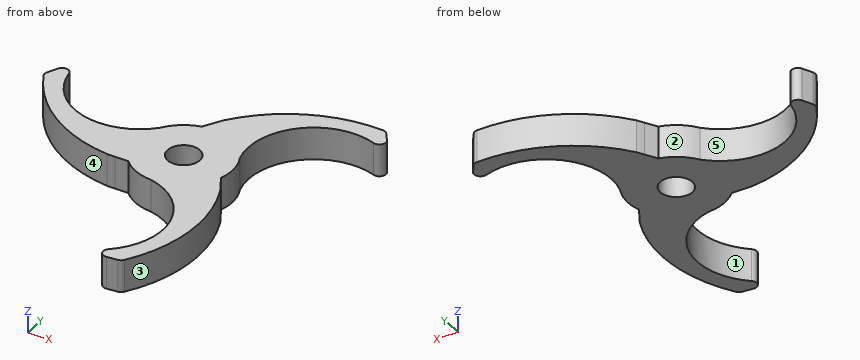
Autodesk Inventor part; units mm, degrees
ref_plane "Work Plane3" through (0, 0, 5) normal (0, 0, -1) x (-1, 0, 0)
ref_plane "YZ Plane" through (0, 0, 0) normal (1, 0, 0) x (0, 1, 0)
ref_plane "XZ Plane" through (0, 0, 0) normal (0, 1, 0) x (-1, 0, 0)
sketch "Sketch1" plane through (0, 0, 0) normal (0, 0, 1) x (1, 0, 0)
  circle A0 centre (0, 0) radius 15
  circle A1 centre (0, 0) radius 55
  line L0 (15, 0) -> (55, 0) construction
  circle A2 centre (35, 0) radius 20 construction
  circle A3 centre (-17.5, 30.3109) radius 20 construction
  circle A4 centre (-17.5, -30.3109) radius 20 construction
  line L1 (0, 0) -> (-10.834, 10.3742)
  line L2 (0, 0) -> (27.5, -47.6314)
  line L3 (0, 0) -> (-55, 0) construction
  line L4 (0, 0) -> (27.5, 47.6314)
  line L5 (17.5, 30.3109) -> (27.5, 47.6314) construction
  line L6 (-1.4324, 18.1475) -> (18.5676, 52.7885) construction
  line L7 (18.5676, 52.7885) -> (36.4324, 42.4743) construction
  line L8 (36.4324, 42.4743) -> (16.4324, 7.8333) construction
  line L9 (16.4324, 7.8333) -> (-1.4324, 18.1475) construction
  line L10 (-1.4324, 18.1475) -> (36.4324, 42.4743) construction
  line L11 (18.5676, 52.7885) -> (16.4324, 7.8333) construction
  line L12 (-1.4891, -18.1802) -> (18.5109, -52.8212) construction
  line L13 (18.5109, -52.8212) -> (36.4891, -42.4416) construction
  line L14 (36.4891, -42.4416) -> (16.4891, -7.8006) construction
  line L15 (16.4891, -7.8006) -> (-1.4891, -18.1802) construction
  line L16 (-1.4891, -18.1802) -> (36.4891, -42.4416) construction
  line L17 (18.5109, -52.8212) -> (16.4891, -7.8006) construction
  line L18 (-55.0081, 10.3109) -> (-15, 10.3109) construction
  line L19 (-15, 10.3109) -> (-15, -10.3109) construction
  line L20 (-15, -10.3109) -> (-55.0081, -10.3109) construction
  line L21 (-55.0081, -10.3109) -> (-55.0081, 10.3109)
  line L22 (-55.0081, 10.3109) -> (-15, -10.3109) construction
  line L23 (-15, 10.3109) -> (-55.0081, -10.3109) construction
  line L24 (-39.1178, -2.5) -> (-30.8902, -2.5) construction
  line L25 (-30.8902, -2.5) -> (-30.8902, 2.5) construction
  line L26 (-30.8902, 2.5) -> (-39.1178, 2.5) construction
  line L27 (-39.1178, 2.5) -> (-39.1178, -2.5) construction
  line L28 (-39.1178, -2.5) -> (-30.8902, 2.5) construction
  line L29 (-30.8902, -2.5) -> (-39.1178, 2.5) construction
  line L30 (-55.0081, 10.3109) -> (-55.0081, -10.3109) construction
  line L31 (-55.0081, 10.3109) -> (-55.0081, -10.3109) construction
  circle A5 centre (0, 0) radius 5
  arc A6 (-47.6318, 23.7685) -> (-10.834, 10.3742) centre (-27.4698, 21.9149) ccw
  line L32 (-15, -10.3109) -> (-10.8943, -10.3109)
  line L33 (-46.714, 28.5112) -> (-52.5923, 15.6119)
  arc A7 (-52.5567, 13.8792) -> (-17.5, -10.3109) centre (-12.7886, 34.0144) ccw
  arc A8 (-17.5, -10.3109) -> (-15, -10.3109) centre (-16.25, 36.3845) ccw
  arc A9 (-52.5923, 15.6119) -> (-52.5567, 13.8792) centre (-50.7724, 14.7826) ccw
  line L34 (-46.714, 28.5112) -> (-45.8939, 30.3109)
  arc A10 (-45.8939, 30.3109) -> (-47.6318, 23.7685) centre (-27.4698, 21.9149) ccw
  arc A11 (14.2587, -52.455) -> (17.6795, -10) centre (-23.063, -28.0825) ccw
  arc A12 (12.7758, -53.3523) -> (14.2587, -52.455) centre (12.5841, -51.3615) ccw
  line L35 (-1.3344, -54.7111) -> (12.7758, -53.3523)
  arc A13 (3.2318, -53.1346) -> (-3.5673, -14.5696) centre (-5.2439, -34.747) ccw
  arc A14 (-3.3031, -54.9007) -> (3.2318, -53.1346) centre (-5.2439, -34.747) ccw
  line L36 (-1.3344, -54.7111) -> (-3.3031, -54.9007)
  line L37 (16.4295, -7.8349) -> (14.3766, -4.2793)
  arc A15 (17.6795, -10) -> (16.4295, -7.8349) centre (-23.3849, -32.2652) ccw
  circle A16 centre (0, 0) radius 15
  arc A17 (38.2981, 38.5759) -> (-0.1795, 20.3109) centre (35.8517, -5.9319) ccw
  arc A18 (39.8165, 37.7403) -> (38.2981, 38.5759) centre (38.1883, 36.5789) ccw
  line L38 (48.0484, 26.2) -> (39.8165, 37.7403)
  arc A19 (44.4, 29.3661) -> (14.4013, 4.1954) centre (32.7138, 12.8321) ccw
  arc A20 (49.1969, 24.5898) -> (44.4, 29.3661) centre (32.7138, 12.8321) ccw
  line L39 (48.0484, 26.2) -> (49.1969, 24.5898)
  line L40 (-1.4295, 18.1458) -> (-3.4823, 14.5902)
  arc A21 (-0.1795, 20.3109) -> (-1.4295, 18.1458) centre (39.6349, -4.1193) ccw
  circle A22 centre (0, 0) radius 15
  point P0 (-27.5, 47.6314)
  point P1 (-27.5, -47.6314)
  point P2 (17.5, -30.3109)
  point P3 (-35.004, 0)
  point P4 (-52.9855, 14.7493)
  point P5 (-52.9855, 14.7493)
  point P6 (7.5, -12.9904)
  point P7 (-12.5218, 8.2586)
  point P8 (-7.5, 12.9904)
  point P9 (-7.5, -12.9904)
  point P10 (-0.8912, -14.9735)
  point P11 (13.413, 6.7149)
  dimension "d0" = 30
  dimension "d1" = 40
  dimension "d4" = 360
  dimension "d6" = 5
  dimension "d11" = 10
  dimension "d24" = 2
  dimension "d31" = 360
extrude "Extrusion1" add sketch "Sketch1" along normal blind 10 contours A0 L2 A5 L4 A19 | A19 A0 | L37 A15 A11 L2 A0 | A0 L4 A17 A18 L38 L39 A20 A19 | L2 A11 A12 L35 L36 A14 A13 A0 | A0 A13 A6 L1 A5 L2 | L4 A5 L1 A0 | A0 L40 A21 A17 L4 | A0 A13 | A6 A0 | L32 A8 A7 A9 L33 L34 A10 A6 A0
fillet "Fillet1" radius 2 3 edges at (-45.8939, 30.3109, 5) (49.1969, 24.5898, 5) (-3.3031, -54.9007, 5)
sketch "Sketch2" plane through (0, 0, 10) normal (0, 0, 1) x (1, 0, 0)
  line L0 (17.5, 30.3109) -> (27.5, 47.6314) construction
  line L1 (27.5, 47.6314) -> (2.5, 4.3301)
  circle A0 centre (0, 0) radius 5
  circle A1 centre (0, 0) radius 15 construction
  circle A2 centre (0, 0) radius 5 construction
ref_plane "Work Plane3" through (0, 0, 5) normal (0, 0, -1) x (-1, 0, 0)
properties part number "Combine mk5"
Can you work these out from the model? Positions are in its coordinate system, mm. Face numbers are marked on the shaded views. A direction names the side the tool comes from. Give positions to 0.01 mm unless a question says otherwise; leave off trailing zeros. Order: outer loops, then holes, each group sorted by start corner. A loop starts at its lowest first (then second) coordinate and runs counter-clockwise, first axis right, second up. Notation, with made-up numbers: (45, 84) - (82, 84) arc R6 ccw to (82, 88) - close; hole circle Ø3 at (3, -7.75). An arc over 180 degrees is marked (long way). Use a Markdown table: item, result. Add a question column.
Q1. If we section it at C-C on y = -47: Write out the boundary of the cut face in (x, z), plus the area to 3 significant figures.
Q2. I'm going to push flat-ended pins straight in: pin 1 (2 mm diameter, centred on x = -13.5, z = 3, fed in from -Y); pin 2 (5 mm diameter, centred on x = 31, z = 4.5, fed in from -Y); pin 3 (2 mm diameter, centred on x = 19, z = 7.5, fed in from -Y). Where does each tip first touch, or does it pass through?
Q3. Please list where these lines run through material, in increasing order: line 1 along Y through (x, z) = (0, 3.75); line 2 along X through (y, z) = (0.5, 5); line 3 along X through (y, z) = (0, 7).
Q4. If we section it at A-A on y = 0: Write out the boundary of the cut face in (x, z).
Q5. On a 3-axis mill with a long thin cutter (end or side, diameter ignored), from which of +Z, -Z, +X, -X, +Y, -Y can I reach the whole of each face in a straight line? I mean the marked faces 1 and 2. Say none if no direction works.
Q6. If we mould it in two halves opening along Y, with no side actions, what happens to the marked faces 3, 4 and 5? For each: released by +Y, released by -Y, zero draft, split by the parting line, or undercut.
Q7. If we section it at B-B on x = -19: Write out the boundary of the cut face in (y, z).
Answers follow:
| question | item | result |
|---|---|---|
| 1 | outline | (10.87, 0) - (17.3, 0) - (17.3, 10) - (10.87, 10) - close |
| 1 | area | 64.2 mm^2 |
| 2 | pin 1 | stops at y = -10.31 |
| 2 | pin 2 | stops at y = 32.64 |
| 2 | pin 3 | stops at y = -45.42 |
| 3 | line 1 | y = -15.19 to -5, 5 to 20.56 |
| 3 | line 2 | x = -42.18 to -4.97, 4.97 to 14.99 |
| 3 | line 3 | x = -41.6 to -5, 5 to 15 |
| 4 | outline | (-41.6, 0) - (-5, 0) - (-5, 10) - (-41.6, 10) - close; (5, 0) - (15, 0) - (15, 10) - (5, 10) - close |
| 5 | face 1 | +Z, -Z, -X |
| 5 | face 2 | +Z, -Z, +Y |
| 6 | face 3 | undercut |
| 6 | face 4 | released by -Y |
| 6 | face 5 | released by +Y |
| 7 | outline | (-10.13, 0) - (3.52, 0) - (3.52, 10) - (-10.13, 10) - close |
